Geometry: final body of the model. Coordinates: model frame, mm. A direction names the side the tool comes from. Give positions to 0.01 mm unless a question says otherwise; leave off trailing zeros. Write each loop counter-clockwise with the first axis right and the second up, starting at its lowest first coordinate (ties: lowest second). Pieces come first, ordered by that corner, then holes. Notation, with made-up numbers: (13.25, 56) -> (70.25, 56) arc R18 ccw to (70.25, 80) -> close; hole circle Ø7 at (61, 64.25). An arc over 180 degrees is marked (long way). Answer in a Markdown table with one row per item. Add a question column.
Item 1: First-contact query: P1, Ø3, axis at y = 39.5, z = 14, coming from the +X side; P2, Ø5, axis at y = 39, z = 10, coming from the +X side; P3, Ø3, axis at y = 39, z = 12, coming from the +X side. Flat tips, straight axial feed; report the tip coordinate or a pass-through.
Item 2: Section query C-C on x = -5.5. Output: boundary loops of the cut face in (y, z).
Item 3: Access query for faces 4 (the cylindrical face through (-12.21, -32.97, 9.86)), 5 (the cylindrical face through (15, 43, 7)), 6 (the flat face through (-0.75, 42, 8)). Directions: +Z, -Z, +X, -X, +Y, -Y. A direction counts if a zero-diameter tool reaches every point of the face in a straight line with its end or side. Return the directions, or none.
Item 4: Section query A-A on y = 39. Output: boundary loops of the cut face in (x, z), plus the area to 3 significant figures.
Item 5: Draft query along Z for faces 1 (the flat face through (0, 1, 20)), 2 (the flat face through (0.75, 42.3, 9.9)), 3 (the cylindrical face through (5, 42, 10)). Return one class per face: +Z half, -Z half, draft (parallel to the pull), parting line (faces both ways), or undercut.
Item 6: Material intervals for probe 1 along Y at (x, z) = (13.75, 10); probe 2 along Y at (x, z) = (-5.5, 10); probe 3 along Y at (x, z) = (-6.25, 10), sorted ascending. Write a range as from..to.
Item 7: Section query B-B on z = 10. Output: boundary loops of the cut face in (x, y), plus the area to 3 significant figures.
Item 8: Section query D-D on y = 25. Output: boundary loops of the cut face in (x, z), plus the area to 3 significant figures.
```python
from build123d import *

# Parameters (mm, degrees)
CROQUIS1_R              = 3
SALIENTE_EXTRUIR1_DEPTH = 20
CROQUIS2_R              = 3
CORTAR_EXTRUIR1_DEPTH   = 30
CROQUIS3_R              = 5
CORTAR_EXTRUIR2_DEPTH   = 10


with BuildPart() as part:
    # Croquis1 → Saliente-Extruir1 (new body)
    with BuildSketch(Plane.XY):
        with BuildLine():
            Line((-0.75, 34.971835338), (-0.75, 45))
            Line((-0.75, 45), (-20, 45))
            Line((-20, 45), (-20, -45))
            Line((-20, -45), (20, -45))
            Line((20, -45), (20, 45))
            Line((20, 45), (0.75, 45))
            Line((0.75, 45), (0.75, 34.971835338))
            ThreePointArc((0.75, 34.971835338), (0, 15), (-0.75, 34.971835338))
        make_face()
        with Locations((-10, -35)):
            Circle(CROQUIS1_R, mode=Mode.SUBTRACT)
        with Locations((10, -35)):
            Circle(CROQUIS1_R, mode=Mode.SUBTRACT)
    extrude(amount=SALIENTE_EXTRUIR1_DEPTH)

    # Croquis2 → Cortar-Extruir1 (cut)
    with BuildSketch(Plane(origin=(20, 0, 0), x_dir=(0, 0, -1), z_dir=(1, 0, 0))):
        with Locations((-10, 39)):
            Circle(CROQUIS2_R)
    extrude(amount=-CORTAR_EXTRUIR1_DEPTH, mode=Mode.SUBTRACT)

    # Croquis3 → Cortar-Extruir2 (cut)
    with BuildSketch(Plane(origin=(20, 0, 0), x_dir=(0, 0, -1), z_dir=(1, 0, 0))):
        with Locations((-10, 39)):
            Circle(CROQUIS3_R)
    extrude(amount=-CORTAR_EXTRUIR2_DEPTH, mode=Mode.SUBTRACT)


solid = part.part
```
Findings below:
| question | item | result |
|---|---|---|
| 1 | P1 | stops at x = 20 |
| 1 | P2 | stops at x = -10 |
| 1 | P3 | stops at x = 10 |
| 2 | outline | (-45, 0) -> (16.65, 0) -> (16.65, 20) -> (-45, 20) -> close; (33.35, 0) -> (45, 0) -> (45, 20) -> (33.35, 20) -> close; hole circle Ø6 at (39, 10) |
| 3 | face 4 | +Z, -Z |
| 3 | face 5 | +X |
| 3 | face 6 | +Z, -Z, +Y |
| 4 | outline | (-20, 0) -> (-0.75, 0) -> (-0.75, 7) -> (-10, 7) -> (-10, 13) -> (-0.75, 13) -> (-0.75, 20) -> (-20, 20) -> close; (0.75, 0) -> (20, 0) -> (20, 5) -> (10, 5) -> (10, 7) -> (0.75, 7) -> close; (0.75, 13) -> (10, 13) -> (10, 15) -> (20, 15) -> (20, 20) -> (0.75, 20) -> close |
| 4 | area | 559 mm^2 |
| 5 | face 1 | +Z half |
| 5 | face 2 | draft |
| 5 | face 3 | undercut |
| 6 | probe 1 | y = -45..34, 44..45 |
| 6 | probe 2 | y = -45..16.65, 33.35..36, 42..45 |
| 6 | probe 3 | y = -45..17.19, 32.81..36, 42..45 |
| 7 | outline | (-20, -45) -> (20, -45) -> (20, 34) -> (10, 34) -> (10, 36) -> (0.75, 36) -> (0.75, 34.97) arc R10 cw (long way) to (-0.75, 34.97) -> (-0.75, 36) -> (-10, 36) -> (-10, 42) -> (-0.75, 42) -> (-0.75, 45) -> (-20, 45) -> close; (0.75, 42) -> (10, 42) -> (10, 44) -> (20, 44) -> (20, 45) -> (0.75, 45) -> close; hole circle Ø6 at (-10, -35); hole circle Ø6 at (10, -35) |
| 7 | area | 3,000 mm^2 |
| 8 | outline | (-20, 0) -> (-10, 0) -> (-10, 20) -> (-20, 20) -> close; (10, 0) -> (20, 0) -> (20, 20) -> (10, 20) -> close |
| 8 | area | 400 mm^2 |
